The listing builds one solid part. Answer for the finished solid, in the listing's coordinates (mm). A direction names the side the tool comes from. Coordinates: 2 decimals unless noted, no trailing zeros. Order: outer loops, then holes, each group sorted by start corner. A loop starts at its lowest first (then second) coordinate and runs counter-clockwise, first axis right, second up.
Autodesk Inventor part; units mm, degrees
ref_plane "YZ Plane" through (0, 0, 0) normal (1, 0, 0) x (0, 1, 0)
ref_plane "XZ Plane" through (0, 0, 0) normal (0, 1, 0) x (-1, 0, 0)
ref_plane "XY Plane" through (0, 0, 0) normal (0, 0, 1) x (1, 0, 0)
sketch "Sketch1" plane through (0, 0, 0) normal (0, 0, 1) x (1, 0, 0)
  line L0 (0, 0) -> (25, 0)
  line L1 (25, 0) -> (25, 30.6)
  line L2 (25, 30.6) -> (0, 30.6)
  line L3 (0, 30.6) -> (0, 0)
  dimension "d0" = 25
  dimension "d1" = 30.6
extrude "Extrusion1" add sketch "Sketch1" along normal blind 10
sketch "Sketch2" plane through (0, 0, 10) normal (0, 0, 1) x (1, 0, 0)
  circle A0 centre (12.5, 15.3) radius 10
  line L0 (25, 0) -> (25, 30.6)
  line L1 (0, 0) -> (25, 0)
  dimension "d4" = 12.5
  dimension "d6" = 20
  dimension "d19" = 15.3
extrude "Extrusion2" add sketch "Sketch2" along normal blind 100
sketch "Sketch3" plane through (0, 0, 0) normal (0, 0, -1) x (-1, 0, 0)
  circle A0 centre (-12.5, 5.8) radius 3
  circle A1 centre (-12.5, 24.8) radius 3
  line L0 (0, 30.6) -> (0, 0)
  line L1 (0, 0) -> (-25, 0)
  point P0 (-12.5, 0)
  dimension "d9" = 6
  dimension "d10" = 6
  dimension "d11" = 12.5
  dimension "d12" = 12.5
  dimension "d13" = 19
  dimension "d14" = 5.8
extrude "Extrusion3" cut sketch "Sketch3" against normal blind 20
sketch "Sketch4" plane through (0, 0, 10) normal (0, 0, 1) x (1, 0, 0)
  arc A0 (9.5003, 5.7605) -> (15.4997, 5.7605) centre (12.5, 5.8) ccw
  circle A1 centre (12.5, 5.8) radius 5
  arc A2 (15.4997, 24.8395) -> (9.5003, 24.8395) centre (12.5, 24.8) ccw
  circle A3 centre (12.5, 24.8) radius 5
  point P0 (0, 0)
  dimension "d17" = 10
  dimension "d18" = 10
extrude "Extrusion4" cut sketch "Sketch4" along normal blind 37
properties part number "handle_vertical"
1) Section B-B (y = 15.3) is taken. Give the vertices of the cut face in (x, z), then the cut area to 3 significant figures.
2) Section A-A (x = 12.5) is taken. Give the vertices of the cut face in (y, z), then the cut area to 3 significant figures.
3) Section D-D (x = 1.5) is taken. Give the vertices of the cut face in (y, z), then the cut area to 3 significant figures.
4) Determine the mould class of faces 5 (the face through (0, 16, 5)), 6 (the face through (25, 15, 5)), 7 (the face through (12, 8, 47)) for opening direction X: released by +X, released by -X, zero draft, split by the parting line, or undercut.
5) Section C-C (z = 100.5) is taken. Give the vertices of the cut face in (x, y).
6) A tool of negligible diameter and unlimited length cuts with its end or side. For faces 1 (the face through (12.4, 10.8, 28.2)), 2 (the face through (14.9, 23, 4.9)), 3 (the face through (12, 23, 47)), 4 (the face through (11.198, 5.385, 59.3)), from which of +Z, -Z, +X, -X, +Y, -Y can it reach the whole face along a straight path? Write none if from no direction.
7) Consider L1, parallel to Y at x = 12.5, z = 2.75; L2, parallel to Z at x = 14.25, y = 20.5; L3, parallel to X at y = 9, z = 39.5. Determine where each line is inside the solid, lowest interval first.
8) Each of these flat-tipped pins is pushed along its axis until it touches: P1, Ø12, axis at x = 4.5, z = 90, coming from the -Y side; P2, Ø10, axis at x = 22.5, z = 25.5, coming from the -Y side; P3, Ø8, axis at x = 5.5, z = 52, coming from the +Y side. Where does it stop, or does it pass through?
Filled sheet:
1. outline: (0, 0) - (25, 0) - (25, 10) - (22.5, 10) - (22.5, 110) - (2.5, 110) - (2.5, 10) - (0, 10) - close
1. area: 2,250 mm2
2. outline: (0, 0) - (2.8, 0) - (2.8, 10) - (0, 10) - close; (5.3, 47) - (10.8, 47) - (10.8, 10) - (8.8, 10) - (8.8, 0) - (21.8, 0) - (21.8, 10) - (19.8, 10) - (19.8, 47) - (25.3, 47) - (25.3, 110) - (5.3, 110) - close; (27.8, 0) - (30.6, 0) - (30.6, 10) - (27.8, 10) - close
2. area: 1,780 mm2
3. outline: (0, 0) - (30.6, 0) - (30.6, 10) - (0, 10) - close
3. area: 306 mm2
4. face 5: released by -X
4. face 6: released by +X
4. face 7: undercut
5. outline: circle Ø20 at (12.5, 15.3)
6. face 1: -Y
6. face 2: -Z
6. face 3: +Y
6. face 4: +Z
7. L1: y = 0 to 2.8, 8.8 to 21.8, 27.8 to 30.6
7. L2: z = 0 to 10, 47 to 110
7. L3: x = 4.73 to 8.66, 16.34 to 20.27
8. P1: stops at y = 5.5
8. P2: stops at y = 6.64
8. P3: stops at y = 24.84
